Check sheet for the modelled part. Datum: model origin and axes. Units: mm. Round coordinates to 2 decimals unless told otherwise and drop trailing zeros. Write each loop counter-clockwise with the first axis right and the second up, starting at its lowest first coordinate (ties: lowest second). Pieces come first, ordered by that corner, then holes. Notation, with made-up numbers: M 2,31.5 L 51,31.5 A24 cw 51,42.5 Z; hole C 2.5,28.5 d2. An arc over 180 degrees is marked long. Answer in a Markdown table with one row per item.
Autodesk Inventor part; units mm, degrees
ref_plane "YZ Plane" through (0, 0, 0) normal (1, 0, 0) x (0, 1, 0)
ref_plane "XZ Plane" through (0, 0, 0) normal (0, 1, 0) x (-1, 0, 0)
ref_plane "XY Plane" through (0, 0, 0) normal (0, 0, 1) x (1, 0, 0)
sketch "Sketch1" plane through (0, 0, 0) normal (0, 0, 1) x (1, 0, 0)
  line L0 (0, 0) -> (-13.73, 0)
  line L1 (-13.73, 0) -> (-13.73, -17)
  arc A0 (-34.11, -61.5) -> (-13.73, -17) centre (-72.5032, -17) ccw
  arc A1 (-34.11, -61.5) -> (-54.49, -106) centre (4.2832, -106) ccw
  line L2 (-54.49, -106) -> (-54.49, -246.2)
  line L3 (-54.49, -246.2) -> (-42.6683, -297)
  line L4 (-42.6683, -297) -> (0, -297)
  line L5 (0, -297) -> (0, 0)
  line L6 (0, -356.4) -> (0, 59.4)
  dimension "d0" = 13.73
  dimension "d1" = 17
  dimension "d2" = 54.49
  dimension "d3" = 106
  dimension "d4" = 13.1
  dimension "d5" = 297
  dimension "d6" = 50.8
revolve "Revolution1" add sketch "Sketch1" angle 360 about axis through (0, -10, 0) along (0, 1, 0)
shell "Shell1" thickness 0.5 removed faces 1 at (0.5517, 0, -4.0152)
sketch "Sketch2" plane through (0, 0, 0) normal (0, 0, 1) x (1, 0, 0)
  line L0 (53.99, -106) -> (-53.99, -106)
  line L1 (13.73, 0) -> (-13.73, 0) construction
  line L2 (-53.99, 0) -> (53.99, 0)
  line L3 (53.99, 0) -> (53.99, -46)
  line L4 (53.99, -46) -> (-53.99, -46)
  line L5 (-53.99, -46) -> (-53.99, 0)
  line L6 (53.99, -266.2) -> (-53.99, -266.2)
  line L7 (-53.99, -266.2) -> (-53.99, -297)
  line L8 (-53.99, -297) -> (53.99, -297)
  line L9 (53.99, -297) -> (53.99, -266.2)
  line L10 (42.6683, -297) -> (-42.6683, -297)
  line L11 (54.49, -246.2) -> (-54.49, -246.2)
  point P0 (0, 0)
  dimension "d10" = 60
  dimension "d11" = 20
extrude "circumferentialCuts" cut sketch "Sketch2" along normal through all both and the other way through all
sketch "Sketch3" plane through (0, 0, 0) normal (0, 0, 1) x (1, 0, 0)
  line L0 (-0.5, 0) -> (0.5, 0)
  line L1 (0.5, 0) -> (0.5, -266.2)
  line L2 (0.5, -266.2) -> (-0.5, -266.2)
  line L3 (-0.5, -266.2) -> (-0.5, 0)
  line L4 (49.8358, -266.2) -> (-49.8358, -266.2)
  point P0 (0, 0)
  point P1 (0, 0)
  dimension "d15" = 1
extrude "vertical" cut sketch "Sketch3" against normal through all
sketch "Sketch4" plane through (340.0931, -246.1426, -50.8714) normal (-0.0092, 0, 1) x (1, 0, 0.0092)
  line L0 (-31, 200.1426) -> (-30, 200.1426)
  line L1 (-30, 200.1426) -> (-30, 30)
  line L2 (-30, 30) -> (-31, 30)
  line L3 (-31, 30) -> (-31, 200.1426)
  line L4 (-309.6074, 200.1426) -> (-308.6074, 200.1426)
  line L5 (-308.6074, 200.1426) -> (-308.6074, 30)
  line L6 (-308.6074, 30) -> (-309.6074, 30)
  line L7 (-309.6074, 30) -> (-309.6074, 200.1426)
  line L8 (-0.8007, 200.1426) -> (-338.8067, 200.1426)
  line L9 (0, 0) -> (0, 140.1426)
  line L10 (0, 0) -> (-339.6074, 0)
  line L11 (-339.6074, 140.1426) -> (-339.6074, 0)
  dimension "d18" = 1
  dimension "d19" = 30
  dimension "d20" = 30
  dimension "d21" = 30
sketch "Sketch16" plane through (340.1023, -246.2, -51.3714) normal (0.0092, 0, -1) x (-1, 0, -0.0092)
  line L0 (0, 1) -> (30.0046, 31.0046)
  line L1 (30.0046, 30.0574) -> (30.0046, 140.2)
  line L2 (0, 140.2) -> (0, 0)
  point P0 (339.6166, 246.2)
  dimension "d87" = 45
  dimension "d88" = 1
sketch "Sketch23" plane through (0.5, -246.2, -54.4877) normal (0.0092, 0, -1) x (-1, 0, -0.0092)
  line L0 (0, 1) -> (-30.0046, 31.0046)
  line L1 (0, 0) -> (0, 140.2)
  line L2 (-30.0046, 140.2) -> (-30.0046, 30.0574)
  line L3 (-339.6166, 0) -> (0, 0)
  point P0 (0, 246.2)
  dimension "d136" = 45
  dimension "d137" = 1
sketch "Sketch17" plane through (202.4892, -243.6006, -50.6341) normal (-0.0092, 0, 1) x (1, 0, 0.0092)
  line L0 (105.596, 0) -> (105.596, 30.0046)
  line L1 (105.9965, 30.0046) -> (0, 30.0046)
  line L2 (0, 0) -> (136.0011, 0)
  line L3 (106.596, 27.458) -> (106.596, 137.6006)
  point P0 (-202.016, 243.6006)
  dimension "d101" = 1
sketch "Sketch24" plane through (2.081, -243.6006, -52.4731) normal (-0.0092, 0, 1) x (1, 0, 0.0092)
  line L0 (31.0046, 30.0046) -> (31.0046, 0)
  line L1 (-1.5994, 0) -> (136.0011, 0)
  line L2 (136.0011, 30.0046) -> (28.4052, 30.0046)
  point P0 (-1.5994, 243.6006)
  point P1 (0, 0)
  point P2 (136.0011, 0)
  point P3 (30.0046, 30.0046)
  point P4 (-1.5994, -2.5994)
  point P5 (28.4052, 27.458)
  dimension "d138" = 1
equation "\"d13\" = Thickness"
equation "\"d16\" = Thickness"
equation "\"BendRadius\" = Thickness"
equation "\"BendReliefWidth\" = Thickness"
equation "\"BendReliefDepth\" = 0.5 * Thickness"
equation "\"CornerReliefSize\" = 4 * Thickness"
equation "\"MinimumRemnant\" = 2 * Thickness"
equation "\"TransitionRadius\" = BendRadius"
equation "\"JacobiRadiusSize\" = BendRadius"
equation "\"GapSize\" = Thickness"
properties material "PET Plastic"
1. Scan lines: L1, parallel to X at y = -148, z = 0; L2, parallel to X at y = -90.5, z = -22.5; L3, parallel to Z at x = 0, y = -151.5. Record each from-to range of solid material in increasing order.
Found:
| item | result |
|---|---|
| L1 | x = -54.49 to -53.99, 53.99 to 54.49 |
| L2 | x = -47.33 to -46.76, 46.76 to 47.33 |
| L3 | z = 53.99 to 54.49 |
2. Go/stop test with flat-tipped pins: pin 1 (17 mm diameter, centred on y = -122, z = -30, fed in from +X); pin 2 (2 mm diameter, centred on x = 18.5, z = -34.5, fed in from -Y); pin 3 (6 mm diameter, centred on y = -166, z = 43.5, fed in from +X). Record where each tip stops, or that it passes through.
Found:
| item | result |
|---|---|
| pin 1 | stops at x = 50.07 |
| pin 2 | stops at y = -68.29 |
| pin 3 | stops at x = 36.45 |
3. Section check A-A, the plane y = -138.5. Record the cut outline in (x, z).
Found:
| item | result |
|---|---|
| outline | M -0.5,-54.49 L -0.5,-53.99 A53.99 cw long 0.5,-53.99 L 0.5,-54.49 A54.49 ccw long Z |
